Check sheet for the modelled part. Datum: model origin and axes. Units: mm. A direction names the side the tool comes from. Round coordinates to 2 decimals unless told otherwise and drop trailing zeros. Loops run counter-clockwise (first coordinate to the right, second up) from the corner with the lowest first, then second, coordinate; pieces in that order, holes last. Notation, with made-up numbers: (65, 87) -> (122, 87) arc R21 cw to (122, 104) -> close; hole circle Ø7 at (-20.75, 42). An arc over 180 degrees is marked (long way). Return JSON: item names as keys, results as strings.
from build123d import *

# Parameters (mm, degrees)
F0_R     = 1
F1_DEPTH = 3.475
F2_DEPTH = 2.25
F4_DEPTH = 1.5
F6_DEPTH = 1.5


with BuildPart() as f1:
    # F0 (on Front) → F1 (new body, symmetric)
    with BuildSketch(Plane.XZ):
        with BuildLine():
            Line((0, 3.7288318854), (0, 0))
            Line((0, 0), (6.9967252202, 0))
            add(Edge.make_bspline(
                [(6.9967252202, 0), (9.2797642574, -4.5221908949), (10.1809287444, -15.1755161159), (7.2002517991, -21.5603647329)],
                knots=[0, 0, 0, 0, 21.5613253416, 21.5613253416, 21.5613253416, 21.5613253416], degree=3))
            add(Edge.make_bspline(
                [(7.2002517991, -21.5603647329), (6.6914390773, -23.4825400211), (8.3887010693, -26.9248684867), (9.7404803961, -26.8961938314)],
                knots=[0, 0, 0, 0, 5.9096390324, 5.9096390324, 5.9096390324, 5.9096390324], degree=3))
            Line((9.7404803961, -26.8961938314), (36.2628367926, -26.5350107441))
            add(Edge.make_bspline(
                [(38.6619754136, -22.4225856364), (38.6969335377, -22.7146428078), (37.0609843214, -26.4885407062), (36.2628367926, -26.5350107441)],
                knots=[0, 0, 0, 0, 4.7610824808, 4.7610824808, 4.7610824808, 4.7610824808], degree=3))
            Line((38.6619754136, -22.4225856364), (37.7328934056, -19.8724068204))
            Line((37.7328934056, -19.8724068204), (36.9564835581, -17.741288223))
            Line((36.9564835581, -17.741288223), (29.1344821453, 3.7288318854))
            add(Edge.make_bspline(
                [(6.9949179888, 3.7288318854), (17.3287056386, 23.4605930746), (26.8724299967, 11.955557391), (29.1344821453, 3.7288318854)],
                knots=[0, 0, 0, 0, 22.1395641565, 22.1395641565, 22.1395641565, 22.1395641565], degree=3))
            Line((6.9949179888, 3.7288318854), (0, 3.7288318854))
        make_face()
        with BuildLine():
            add(Edge.make_bspline(
                [(9.4467252202, 0), (10.9906066209, -2.3621518631), (11.8817396227, -11.8382899378), (11.3527391163, -15.8558540684), (10.8528801655, -18.2185956272)],
                knots=[0, 0, 0, 0, 0.5622964622, 1, 1, 1, 1], degree=3))
            Line((9.4467252202, 0), (26.4606260202, 0))
            Line((26.4606260202, 0), (35.2483888837, -24.1209780218))
            Line((35.2483888837, -24.1209780218), (32.2012024882, -24.1209780218))
            Line((32.2012024882, -24.1209780218), (11.8752977761, -24.1209780218))
            add(Edge.make_bspline(
                [(10.8528801655, -18.2185956272), (10.6736963888, -19.4107137837), (10.0184677383, -20.6313388233), (10.7373066785, -24.130475951), (11.8752977761, -24.1209780218)],
                knots=[0, 0, 0, 0, 0.4837506013, 1, 1, 1, 1], degree=3))
        make_face(mode=Mode.SUBTRACT)
        with Locations((19.8225565255, 11.1334240064)):
            Circle(F0_R, mode=Mode.SUBTRACT)
        with BuildLine():
            Line((26.4606260202, 0), (9.4467252202, 0))
            add(Edge.make_bspline(
                [(9.4467252202, 0), (10.9906066209, -2.3621518631), (11.8817396227, -11.8382899378), (11.3527391163, -15.8558540684), (10.8528801655, -18.2185956272)],
                knots=[0, 0, 0, 0, 0.5622964622, 1, 1, 1, 1], degree=3))
            add(Edge.make_bspline(
                [(10.8528801655, -18.2185956272), (10.6736963888, -19.4107137837), (10.0184677383, -20.6313388233), (10.7373066785, -24.130475951), (11.8752977761, -24.1209780218)],
                knots=[0, 0, 0, 0, 0.4837506013, 1, 1, 1, 1], degree=3))
            Line((11.8752977761, -24.1209780218), (32.2012024882, -24.1209780218))
            Line((32.2012024882, -24.1209780218), (35.2483888837, -24.1209780218))
            Line((35.2483888837, -24.1209780218), (26.4606260202, 0))
        make_face()
    extrude(amount=F1_DEPTH, both=True)

    # F0 (on Front) → F2 (join, symmetric)
    with BuildSketch(Plane.XZ):
        Polygon((38.5574395408, -16.9160417945), (36.9564835581, -17.741288223), (37.7328934056, -19.8724068204), (39.5883468265, -18.9159743354), align=None)
        Polygon((39.5883468265, -18.9159743354), (37.7328934056, -19.8724068204), (38.6619754136, -22.4225856364), (40.6192541122, -20.9159068763), align=None)
    extrude(amount=F2_DEPTH, both=True)

    # F3 (on face) → F4 (cut)
    with BuildSketch(Plane.XZ.offset(3.475)):
        with BuildLine():
            Line((26.4228218723, 0.0341487469), (9.4089210724, 0.0341487469))
            add(Edge.make_bspline(
                [(9.4089210724, 0.0341487469), (10.9528024731, -2.3280031162), (11.8439354748, -11.804141191), (11.3149349685, -15.8217053215), (10.8150760177, -18.1844468803)],
                knots=[0, 0, 0, 0, 0.5622964622, 1, 1, 1, 1], degree=3))
            add(Edge.make_bspline(
                [(10.8150760177, -18.1844468803), (10.635892241, -19.3765650368), (9.9806635904, -20.5971900764), (10.6995025306, -24.0963272041), (11.8374936283, -24.0868292749)],
                knots=[0, 0, 0, 0, 0.4837506013, 1, 1, 1, 1], degree=3))
            Line((11.8374936283, -24.0868292749), (32.1633983403, -24.0868292749))
            Line((32.1633983403, -24.0868292749), (35.2105847359, -24.0868292749))
            Line((35.2105847359, -24.0868292749), (26.4228218723, 0.0341487469))
        make_face()
    extrude(amount=-F4_DEPTH, mode=Mode.SUBTRACT)

    # F5 (on face) → F6 (cut)
    with BuildSketch(Plane(origin=(0, 3.475, 0), x_dir=(-1, 0, 0), z_dir=(0, 1, 0))):
        with BuildLine():
            Line((-26.3866665531, -0.0262773244), (-35.1744294167, -24.1472553462))
            Line((-35.1744294167, -24.1472553462), (-32.1272430211, -24.1472553462))
            Line((-32.1272430211, -24.1472553462), (-11.8013383091, -24.1472553462))
            add(Edge.make_bspline(
                [(-10.7789206985, -18.2448729516), (-10.5997369218, -19.4369911081), (-9.9445082712, -20.6576161477), (-10.6633472114, -24.1567532754), (-11.8013383091, -24.1472553462)],
                knots=[0, 0, 0, 0, 0.4837506013, 1, 1, 1, 1], degree=3))
            add(Edge.make_bspline(
                [(-9.3727657532, -0.0262773244), (-10.9166471538, -2.3884291875), (-11.8077801556, -11.8645672622), (-11.2787796492, -15.8821313928), (-10.7789206985, -18.2448729516)],
                knots=[0, 0, 0, 0, 0.5622964622, 1, 1, 1, 1], degree=3))
            Line((-9.3727657532, -0.0262773244), (-26.3866665531, -0.0262773244))
        make_face()
    extrude(amount=-F6_DEPTH, mode=Mode.SUBTRACT)


solid = f1.part
Q1. Go/stop test with flat-tipped pins: pin 1 (1.5 mm diameter, centred on x = 18.5, z = -4, fed in from -Y) (3 decimals); pin 2 (1.5 mm diameter, centred on x = 28, y = -2.5, fed in from +Z); pin 3 (0.8 mm diameter, centred on x = 21.5, y = 3, fed in from +Z). Record where each tip stops, or that it passes through.
Results list:
{"pin 1": "y = -1.975", "pin 2": "z = 8.28", "pin 3": "z = 14.21"}
Q2. Section check B-B (y = -3). Count the separate pieces of the cut face and the enclosed holes in it, then the cut area to 3 significant figures.
Results list:
{"separate pieces": "1", "enclosed holes": "2", "area": "510 mm^2"}
Q3. Section check A-A (x = 31). Record the boundary of the cut face in (y, z) (3 decimals).
Results list:
{"outline": "(-3.475, -26.607) -> (3.475, -26.607) -> (3.475, -24.147) -> (1.975, -24.147) -> (1.975, -12.689) -> (3.475, -12.689) -> (3.475, -1.392) -> (-3.475, -1.392) -> (-3.475, -12.529) -> (-1.975, -12.529) -> (-1.975, -24.087) -> (-3.475, -24.087) -> close"}
Q4. Draft check along X on faces 6 (the flat face through (22.1, -3.475, 0.3)), 7 (the flat face through (0, 0, 2)), 8 (the flat face through (24, 3, -24.147)). Enter one of: released by +X, released by -X, zero draft, split by the parting line, or undercut.
Results list:
{"face 6": "zero draft", "face 7": "released by -X", "face 8": "undercut"}
Q5. Material ranges on line 1 (Y direction, x = 16.5, z = -3.5) (3 decimals); line 2 (Z direction, x = 6.5, y = 1); line 3 (X direction, y = 2.5, z = -19), recorded low to high.
Results list:
{"line 1": "-1.975 to 1.975", "line 2": "0 to 3.73", "line 3": "8.14 to 10.64, 33.3 to 37.42"}
Q6. Tool access check on faces 1 (the flat face through (39, 2.25, -20)), 2 (the flat face through (37.77, -0.03, -17.32)), 3 (the flat face through (3, 0, 0)), 4 (the flat face through (18, -3, 0.034)), 5 (the flat face through (4, 0, 3.729)). Record the directions out of +Z, -Z, +X, -X, +Y, -Y that give a thin tool (end or side, any length) a straight path to the whole face; none if there is none.
Results list:
{"face 1": "+Z, +X, +Y", "face 2": "+Z, +Y, -Y", "face 3": "-Z, -X, +Y, -Y", "face 4": "-Y", "face 5": "+Z, -X, +Y, -Y"}
